from build123d import *

# Parameters (mm, degrees)
F1_DEPTH = 20
F2_R     = 3
F3_DEPTH = 13
F5_D     = 4.4
F7_D     = 3.3
F7_DEPTH = 6
F7_TIP   = 0.9914200214


with BuildPart() as f1:
    # F0 (on Front) → F1 (new body)
    with BuildSketch(Plane.XZ):
        Polygon((6, -3.4641016151), (6, 3.4641016151), (0, 6.9282032303), (-6, 3.4641016151), (-6, -3.4641016151), (0, -6.9282032303), align=None)
    extrude(amount=F1_DEPTH)

    # F2 (on face) → F3 (cut)
    with BuildSketch(Plane(origin=(0, 0, 0), x_dir=(-1, 0, 0), z_dir=(0, 1, 0))):
        Circle(F2_R)
    extrude(amount=-F3_DEPTH, mode=Mode.SUBTRACT)

    # F5 (through all)
    with Locations(Plane.XZ.offset(20)):
        with Locations((0, 0)):
            Hole(F5_D / 2)

    # F7
    with Locations(Plane.YZ.offset(6)):
        with Locations((-2.75, 0), (-7.25, 0)):
            Hole(F7_D / 2, depth=F7_DEPTH)
            with Locations((0, 0, -(F7_DEPTH + F7_TIP / 2))):  # 118° drill point
                Cone(0, F7_D / 2, F7_TIP, mode=Mode.SUBTRACT)


solid = f1.part
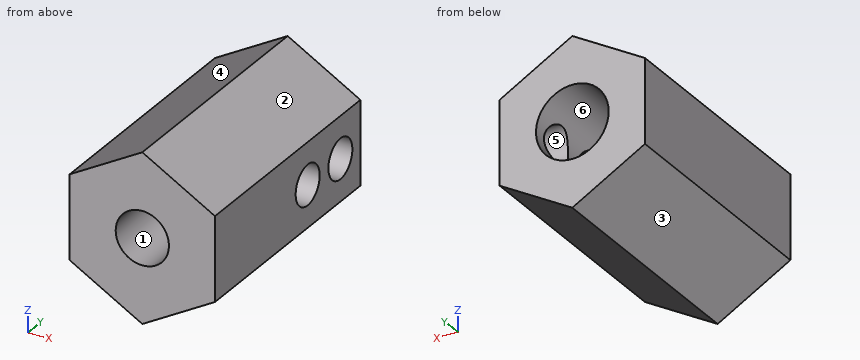
Design review of the part built by this model. Coordinates are the model's own, in mm. Face numbers are marked on the shaded views. A direction names the side the tool comes from. Give positions to 0.01 mm unless a question says otherwise; leave off trailing zeros. Write each loop counter-clockwise with the first axis right and the second up, starting at its lowest first coordinate (ties: lowest second). Pieces come first, ordered by that corner, then holes. Notation, with made-up numbers: M -22.75,61 L 36.25,61 A20 ccw 36.25,77 Z; hole C -37.5,55.25 d8. An arc over 180 degrees is marked long. Answer as a JSON object with one key per item and string values. Group by question number.
1) We need section C-C (x = 1). Give the boundary of the cut face in (y, z).
2) We need section D-D (x = 4.5). Give the boundary of the cut face in (y, z), and give its area (3 significant figures).
3) For line 1 along Y through (x, z) = (3.8, 0); line 2 along Y through (x, z) = (5, -1); line 3 along X through (y, z) = (-3.5, 0), list the stretches that pass through material, from the lowest coordinate up.
4) Clearance check with a flat-ended pin moving along its axis: pin 1 Ø3 at (x, z) = (1, -0.5) entering from +Y. State where the tip first meets the part, or that it passes through.
5) We need section A-A (z = 0). Give the boundary of the cut face in (x, y).
6) Tool access review of the marked faces 4, 5 and 6: name each direction out of +Z, -Z, +X, -X, +Y, -Y from which nothing blocks a thin tool from reaching the whole face with its end or side.
7) We need section B-B (y = -10.5). Give the boundary of the cut face in (x, z).
8) Mouldability with a two-part tool opening along X and no side actions: class the marked faces 1, 2 and 3 as released by +X, released by -X, zero draft, split by the parting line, or undercut.
Answer key:
{
 "1": {"outline": "M -20,-6.35 L 0,-6.35 L 0,-2.83 L -13,-2.83 L -13,-1.96 L -20,-1.96 Z; M -20,1.96 L -13,1.96 L -13,2.83 L 0,2.83 L 0,6.35 L -20,6.35 Z"},
 "2": {"outline": "M -20,-4.33 L 0,-4.33 L 0,4.33 L -20,4.33 Z; hole C -7.25,0 d3.3; hole C -2.75,0 d3.3", "area": "156 mm²"},
 "3": {"line 1": "y = -20 to -8.9, -5.6 to -4.4, -1.1 to 0", "line 2": "y = -20 to -8.56, -5.94 to -4.06, -1.44 to 0", "line 3": "x = -6 to -3"},
 "4": {"pin 1": "stops at y = -13"},
 "5": {"outline": "M -6,-20 L -2.2,-20 L -2.2,-13 L -3,-13 L -3,0 L -6,0 Z; M 2.2,-20 L 6,-20 L 6,-8.9 L 3,-8.9 L 3,-13 L 2.2,-13 Z; M 3,-5.6 L 6,-5.6 L 6,-4.4 L 3,-4.4 Z; M 3,-1.1 L 6,-1.1 L 6,0 L 3,0 Z"},
 "6": {"face 4": "+Z, -X, +Y, -Y", "face 5": "+X", "face 6": "+Y"},
 "7": {"outline": "M -6,-3.46 L 0,-6.93 L 6,-3.46 L 6,3.46 L 0,6.93 L -6,3.46 Z; hole C 0,0 d6"},
 "8": {"face 1": "undercut", "face 2": "released by +X", "face 3": "released by -X"}
}
